```python
from build123d import *

# Parameters (mm, degrees)
SKETCH1_R           = 1.25
SKETCH1_R_2         = 0.75
SKETCH1_W           = 60
SKETCH1_H           = 20
SKETCH1_W_2         = 5
SKETCH1_H_2         = 1
BOSS_EXTRUDE2_DEPTH = 3
SKETCH3_R           = 1.25
CUT_EXTRUDE2_DEPTH  = 3
BOSS_EXTRUDE4_START = -3
SKETCH15_R          = 0.75
BOSS_EXTRUDE4_DEPTH = 3
SKETCH23_R          = 0.75
CUT_EXTRUDE21_DEPTH = 10
SKETCH24_R          = 0.75
CUT_EXTRUDE22_DEPTH = 10
CUT_EXTRUDE23_DEPTH = 10
SKETCH28_W          = 17
SKETCH28_H          = 28
CUT_EXTRUDE25_DEPTH = 3
SKETCH30_R          = 3
CUT_EXTRUDE26_DEPTH = 3
CUT_EXTRUDE28_DEPTH = 3
SKETCH32_R          = 3
CUT_EXTRUDE29_DEPTH = 3
SKETCH33_W          = 10
SKETCH33_H          = 1
CUT_EXTRUDE30_DEPTH = 3
CUT_EXTRUDE32_DEPTH = 3
SKETCH36_R          = 1.5
CUT_EXTRUDE33_DEPTH = 3
SKETCH37_R          = 1.5
CUT_EXTRUDE34_DEPTH = 3
CUT_EXTRUDE36_DEPTH = 3
BOSS_EXTRUDE5_START = -3
SKETCH40_R          = 1.25
BOSS_EXTRUDE5_DEPTH = 3
BOSS_EXTRUDE6_START = -3
SKETCH41_R          = 1.25
BOSS_EXTRUDE6_DEPTH = 3
SKETCH42_R          = 1.5
CUT_EXTRUDE37_DEPTH = 3
SKETCH43_R          = 1.5
CUT_EXTRUDE38_DEPTH = 3
SKETCH44_R          = 1.5
CUT_EXTRUDE39_DEPTH = 3
SKETCH45_R          = 1.5
CUT_EXTRUDE40_DEPTH = 3
SKETCH46_R          = 1.5
CUT_EXTRUDE41_DEPTH = 3
SKETCH47_W          = 20
SKETCH47_H          = 1
CUT_EXTRUDE42_DEPTH = 3
SKETCH48_W          = 11
SKETCH48_H          = 19
CUT_EXTRUDE44_DEPTH = 10


with BuildPart() as part:
    # Sketch1 → Boss-Extrude2 (new body)
    with BuildSketch(Plane.XY):
        Polygon((58.345821786, 13.119852123), (58.345821786, -56.880147877), (-191.654178214, -56.880147877), (-191.654178214, -26.880147877), (-221.654178214, -6.880147877), (-221.654178214, 33.119852123), (-121.654178214, 33.119852123), (-91.654178214, 13.119852123), align=None)
        with Locations((53.345821786, 7.945541925)):
            Circle(SKETCH1_R, mode=Mode.SUBTRACT)
        with Locations((53.345821786, -52.054458075)):
            Circle(SKETCH1_R, mode=Mode.SUBTRACT)
        with Locations((25.505821786, -18.330147877)):
            Circle(SKETCH1_R_2, mode=Mode.SUBTRACT)
        with Locations((-181.654178214, 13.119852123)):
            Rectangle(SKETCH1_W, SKETCH1_H, mode=Mode.SUBTRACT)
        with Locations((25.845821786, 10.619852123)):
            Rectangle(SKETCH1_W_2, SKETCH1_H_2, mode=Mode.SUBTRACT)
        with Locations((40.845821786, 10.619852123)):
            Rectangle(SKETCH1_W_2, SKETCH1_H_2, mode=Mode.SUBTRACT)
    extrude(amount=BOSS_EXTRUDE2_DEPTH)

    # Sketch3 → Cut-Extrude2 (cut)
    with BuildSketch(Plane.XY.offset(3)):
        with Locations((1.345821786, 3.119852123)):
            Circle(SKETCH3_R)
    extrude(amount=-CUT_EXTRUDE2_DEPTH, mode=Mode.SUBTRACT)

    # Sketch15 → Boss-Extrude4 (add)
    with BuildSketch(Plane.XY.offset(3).offset(BOSS_EXTRUDE4_START)):
        with Locations((25.505821786, -18.330147877)):
            Circle(SKETCH15_R)
    extrude(amount=BOSS_EXTRUDE4_DEPTH)

    # Sketch23 → Cut-Extrude21 (cut)
    with BuildSketch(Plane.XY.offset(3)):
        with Locations((-93.524701832, -7.521447448)):
            Circle(SKETCH23_R)
    extrude(amount=-CUT_EXTRUDE21_DEPTH, mode=Mode.SUBTRACT)

    # Sketch24 → Cut-Extrude22 (cut)
    with BuildSketch(Plane.XY.offset(3)):
        with Locations((-107.363654596, -9.638848305)):
            Circle(SKETCH24_R)
    extrude(amount=-CUT_EXTRUDE22_DEPTH, mode=Mode.SUBTRACT)

    # Sketch26 → Cut-Extrude23 (cut)
    with BuildSketch(Plane.XY.offset(3)):
        Polygon((-103.444178214, -47.580147877), (-103.444178214, -42.580147877), (-80.054178214, -2.280147877), (-16.654178214, 13.119852123), (-91.654178214, 13.119852123), (-121.654178214, 33.119852123), (-221.654178214, 33.119852123), (-221.654178214, -6.880147877), (-191.654178214, -26.880147877), (-191.654178214, -56.880147877), (-94.144178214, -56.880147877), align=None)
    extrude(amount=-CUT_EXTRUDE23_DEPTH, mode=Mode.SUBTRACT)

    # Sketch28 → Cut-Extrude25 (cut)
    with BuildSketch(Plane.XY.offset(3)):
        with Locations((-27.554178214, -26.030147877)):
            Rectangle(SKETCH28_W, SKETCH28_H)
        with Locations((-70.554178214, -20.030147877)):
            Rectangle(SKETCH28_W, SKETCH28_H)
    extrude(amount=-CUT_EXTRUDE25_DEPTH, mode=Mode.SUBTRACT)

    # Sketch30 → Cut-Extrude26 (cut)
    with BuildSketch(Plane.XY.offset(3)):
        with Locations((-87.444178214, -42.580147877)):
            Circle(SKETCH30_R)
    extrude(amount=-CUT_EXTRUDE26_DEPTH, mode=Mode.SUBTRACT)

    # Sketch31 → Cut-Extrude28 (cut)
    with BuildSketch(Plane.XY.offset(3)):
        with BuildLine():
            Line((48.345821786, -11.054458075), (48.345821786, -8.054458075))
            Line((48.345821786, -8.054458075), (8.345821786, -8.054458075))
            ThreePointArc((8.345821786, -8.054458075), (4.345821786, -12.054458075), (8.345821786, -16.054458075))
            Line((8.345821786, -16.054458075), (48.345821786, -16.054458075))
            Line((48.345821786, -16.054458075), (48.345821786, -11.054458075))
        make_face()
    extrude(amount=-CUT_EXTRUDE28_DEPTH, mode=Mode.SUBTRACT)

    # Sketch32 → Cut-Extrude29 (cut)
    with BuildSketch(Plane.XY.offset(3)):
        with Locations((1.345821786, 3.119852123)):
            Circle(SKETCH32_R)
    extrude(amount=-CUT_EXTRUDE29_DEPTH, mode=Mode.SUBTRACT)

    # Sketch33 → Cut-Extrude30 (cut)
    with BuildSketch(Plane.XY.offset(3)):
        with Locations((33.345821786, 10.619852123)):
            Rectangle(SKETCH33_W, SKETCH33_H)
    extrude(amount=-CUT_EXTRUDE30_DEPTH, mode=Mode.SUBTRACT)

    # Sketch35 → Cut-Extrude32 (cut)
    with BuildSketch(Plane.XY.offset(3)):
        Polygon((-101.444178214, -45.080147877), (-101.444178214, -39.134230818), (-103.444178214, -42.580147877), (-103.444178214, -47.580147877), (-101.444178214, -49.580147877), align=None)
    extrude(amount=-CUT_EXTRUDE32_DEPTH, mode=Mode.SUBTRACT)

    # Sketch36 → Cut-Extrude33 (cut)
    with BuildSketch(Plane.XY.offset(3)):
        with Locations((-61.654178214, -1.880147877)):
            Circle(SKETCH36_R)
    extrude(amount=-CUT_EXTRUDE33_DEPTH, mode=Mode.SUBTRACT)

    # Sketch37 → Cut-Extrude34 (cut)
    with BuildSketch(Plane.XY.offset(3)):
        with Locations((-87.444178214, -25.580147877)):
            Circle(SKETCH37_R)
    extrude(amount=-CUT_EXTRUDE34_DEPTH, mode=Mode.SUBTRACT)

    # Sketch39 → Cut-Extrude36 (cut)
    with BuildSketch(Plane.XY.offset(3)):
        Polygon((-57.054178214, -20.030147877), (-57.054178214, -56.880147877), (-42.054178214, -56.880147877), (-42.054178214, -1.880147877), (-57.054178214, -1.880147877), align=None)
    extrude(amount=-CUT_EXTRUDE36_DEPTH, mode=Mode.SUBTRACT)

    # Sketch40 → Boss-Extrude5 (add)
    with BuildSketch(Plane.XY.offset(3).offset(BOSS_EXTRUDE5_START)):
        with Locations((53.345821786, 7.945541925)):
            Circle(SKETCH40_R)
    extrude(amount=BOSS_EXTRUDE5_DEPTH)

    # Sketch41 → Boss-Extrude6 (add)
    with BuildSketch(Plane.XY.offset(3).offset(BOSS_EXTRUDE6_START)):
        with Locations((53.345821786, -52.054458075)):
            Circle(SKETCH41_R)
    extrude(amount=BOSS_EXTRUDE6_DEPTH)

    # Sketch42 → Cut-Extrude37 (cut)
    with BuildSketch(Plane.XY.offset(3)):
        with Locations((53.345821786, -51.880147877)):
            Circle(SKETCH42_R)
    extrude(amount=-CUT_EXTRUDE37_DEPTH, mode=Mode.SUBTRACT)

    # Sketch43 → Cut-Extrude38 (cut)
    with BuildSketch(Plane.XY.offset(3)):
        with Locations((-6.654178214, -51.880147877)):
            Circle(SKETCH43_R)
    extrude(amount=-CUT_EXTRUDE38_DEPTH, mode=Mode.SUBTRACT)

    # Sketch44 → Cut-Extrude39 (cut)
    with BuildSketch(Plane.XY.offset(3)):
        with Locations((-61.654178214, -51.880147877)):
            Circle(SKETCH44_R)
    extrude(amount=-CUT_EXTRUDE39_DEPTH, mode=Mode.SUBTRACT)

    # Sketch45 → Cut-Extrude40 (cut)
    with BuildSketch(Plane.XY.offset(3)):
        with Locations((53.345821786, 8.119852123)):
            Circle(SKETCH45_R)
        with Locations((53.345821786, -10.880147877)):
            Circle(SKETCH45_R)
        with Locations((53.345821786, -36.880147877)):
            Circle(SKETCH45_R)
    extrude(amount=-CUT_EXTRUDE40_DEPTH, mode=Mode.SUBTRACT)

    # Sketch46 → Cut-Extrude41 (cut)
    with BuildSketch(Plane.XY.offset(3)):
        with Locations((-16.654178214, 4.119852123)):
            Circle(SKETCH46_R)
    extrude(amount=-CUT_EXTRUDE41_DEPTH, mode=Mode.SUBTRACT)

    # Sketch47 → Cut-Extrude42 (cut)
    with BuildSketch(Plane.XY.offset(3)):
        with Locations((33.345821786, 9.619852123)):
            Rectangle(SKETCH47_W, SKETCH47_H)
    extrude(amount=-CUT_EXTRUDE42_DEPTH, mode=Mode.SUBTRACT)

    # Sketch48 → Cut-Extrude44 (cut)
    with BuildSketch(Plane.XY.offset(3)):
        with Locations((-70.554178214, -43.530147877)):
            Rectangle(SKETCH48_W, SKETCH48_H)
    extrude(amount=-CUT_EXTRUDE44_DEPTH, mode=Mode.SUBTRACT)


solid = part.part
```
Build history of the part. All positions in model axes, mm. A direction names the side the tool comes from. Round coordinates to 2 decimals unless told otherwise and drop trailing zeros. Write each loop counter-clockwise with the first axis right and the second up, starting at its lowest first coordinate (ties: lowest second). Pieces come first, ordered by that corner, then holes. Notation, with made-up numbers: (-26, -22.5) - (-20, -22.5) arc R15 ccw to (-20, -9.5) - close; hole circle Ø1 at (-35.5, -6.5). An arc over 180 degrees is marked (long way). Write each question's results on one line, items separated by ' | '. Start each with the question number.
Item 1: Saw through at A-A (x = 46.5). Write the cut outline in (y, z), and give its area (3 significant figures).
Item 2: Drop flat-ended pins along their axis: P1, Ø4, axis at x = 53.35, y = -10.88, coming from the +Z side; P2, Ø1.5, axis at y = -23, z = 1.5, coming from the -X side. Give the stop position or say it passes through.
Item 3: Saw through at C-C (y = -44). Write the cut outline in (x, z).
Item 4: Mould opens along X. For faces 1 (the face through (-90.9, -20.97, 1.52)), 2 (the face through (48.346, -12, 2)), 3 (the face through (58.346, -21, 1)) say: pulls with the +X half, pulls with the -X half, needs draft (parallel to the pull), parting line crosses it, or undercut.
Item 5: Saw through at B-B (y = -22). Write the cut outline in (x, z).
Item 6: Wall check: L1, parallel to X at y = -48, z = 2.2; L2, parallel to Y at x = 36, z = 2.35; L3, parallel to X at y = -42.5, z = 2.15. Give the ranges that are in metal, low to high. Write a range as [from, to].
Item 7: Saw through at D-D (z = 1.3). State how many separate pieces and enclosed holes the cut face has, and give its area (3 significant figures).
Item 8: Which spindle directions (+Z, -Z, +X, -X, +Y, -Y) get a long thin tool onto all of the face, cutting with end or side? Do faces 4 (the face through (-71, -53.03, 2)), 5 (the face through (-42.054, -30, 2)), 6 (the face through (-97.743, -53.281, 1.521)). Say none if no direction does.
Results are:
1) outline: (-56.88, 0) - (-16.05, 0) - (-16.05, 3) - (-56.88, 3) - close; (-8.05, 0) - (13.12, 0) - (13.12, 3) - (-8.05, 3) - close | area: 186 mm²
2) P1: stops at z = 3 | P2: stops at x = -92.52
3) outline: (-101.44, 0) - (-90.09, 0) - (-90.09, 3) - (-101.44, 3) - close; (-84.8, 0) - (-76.05, 0) - (-76.05, 3) - (-84.8, 3) - close; (-65.05, 0) - (-57.05, 0) - (-57.05, 3) - (-65.05, 3) - close; (-42.05, 0) - (58.35, 0) - (58.35, 3) - (-42.05, 3) - close
4) face 1: pulls with the -X half | face 2: undercut | face 3: pulls with the +X half
5) outline: (-91.5, 0) - (-79.05, 0) - (-79.05, 3) - (-91.5, 3) - close; (-62.05, 0) - (-57.05, 0) - (-57.05, 3) - (-62.05, 3) - close; (-42.05, 0) - (-36.05, 0) - (-36.05, 3) - (-42.05, 3) - close; (-19.05, 0) - (58.35, 0) - (58.35, 3) - (-19.05, 3) - close
6) L1: x = [-101.44, -76.05], [-65.05, -57.05], [-42.05, 58.35] | L2: y = [-56.88, -16.05], [-8.05, 9.12], [11.12, 13.12] | L3: x = [-101.44, -90.44], [-84.45, -76.05], [-65.05, -57.05], [-42.05, 58.35]
7) separate pieces: 1 | enclosed holes: 15 | area: 7,460 mm²
8) face 4: +Z, -Z | face 5: +Z, -Z, -Y | face 6: +Z, -Z, -X, -Y
